```python
from build123d import *

# Parameters (mm, degrees)
SKETCH1_R           = 55
SKETCH1_R_2         = 41.4175
BOSS_EXTRUDE1_DEPTH = 15
CUT_EXTRUDE1_DEPTH  = 80.214897589
CUT_EXTRUDE2_START  = -10
CUT_EXTRUDE2_DEPTH  = 10
SKETCH4_R           = 2.75
CUT_EXTRUDE3_DEPTH  = 84.858511792
FILLET2_R           = 2
CHAMFER2_SIZE       = 1
CHAMFER3_SIZE       = 1


with BuildPart() as part:
    # Sketch1 → Boss-Extrude1 (new body)
    with BuildSketch(Plane(origin=(0, 0, 0), x_dir=(1, 0, 0), z_dir=(0, 1, 0))):
        with Locations(Location((0, 0, 0), (0, 0, 270))):
            Circle(SKETCH1_R)
        with Locations(Location((0, 0, 0), (0, 0, 270))):
            Circle(SKETCH1_R_2, mode=Mode.SUBTRACT)
    extrude(amount=BOSS_EXTRUDE1_DEPTH)

    # Sketch2 → Cut-Extrude1 (cut, through all)
    with BuildSketch(Plane(origin=(0, 15, 0), x_dir=(1, 0, 0), z_dir=(0, 1, 0))):
        with BuildLine():
            Line((-2.5, 41.341979951), (-2.5, 54.94315244))
            ThreePointArc((-2.5, 54.94315244), (0, 55), (2.5, 54.94315244))
            Line((2.5, 54.94315244), (2.5, 41.341979951))
            ThreePointArc((2.5, 41.341979951), (0, 41.4175), (-2.5, 41.341979951))
        make_face()
    extrude(amount=-CUT_EXTRUDE1_DEPTH, mode=Mode.SUBTRACT)

    # Sketch3 → Cut-Extrude2 (cut)
    with BuildSketch(Plane(origin=(0, 15, 0), x_dir=(1, 0, 0), z_dir=(0, 1, 0)).offset(CUT_EXTRUDE2_START)):
        with BuildLine():
            Line((-6.5, 54.614558499), (-6.5, 44.614558499))
            Line((-6.5, 44.614558499), (-32.164284074, 44.614558499))
            ThreePointArc((-32.164284074, 44.614558499), (-19.96826772, 51.247129522), (-6.5, 54.614558499))
        make_face()
        with BuildLine():
            Line((6.5, 44.614558499), (32.164284074, 44.614558499))
            ThreePointArc((32.164284074, 44.614558499), (19.96826772, 51.247129522), (6.5, 54.614558499))
            Line((6.5, 54.614558499), (6.5, 44.614558499))
        make_face()
    extrude(amount=CUT_EXTRUDE2_DEPTH, mode=Mode.SUBTRACT)

    # Sketch4 → Cut-Extrude3 (cut, through all)
    with BuildSketch(Plane.ZY.offset(6.5)):
        with Locations((-49.614558499, 10)):
            Circle(SKETCH4_R)
    extrude(amount=-CUT_EXTRUDE3_DEPTH, mode=Mode.SUBTRACT)

    # Fillet2
    fillet2_edges = [part.edges().sort_by_distance(p)[0] for p in [
        (-19.332142037, 5, -44.614558499),
        (19.332142037, 5, -44.614558499),
    ]]
    fillet(fillet2_edges, radius=FILLET2_R)

    # Chamfer2
    chamfer2_edges = [part.edges().sort_by_distance(p)[0] for p in [
        (0, 0, 55),
        (0, 15, 55),
    ]]
    chamfer(chamfer2_edges, length=CHAMFER2_SIZE)

    # Chamfer3
    chamfer3_edges = [part.edges().sort_by_distance(p)[0] for p in [
        (-41.398615683, 0, 1.250570198),
        (41.398615683, 15, 1.250570198),
    ]]
    chamfer(chamfer3_edges, length=CHAMFER3_SIZE)


solid = part.part
```
Design review of the part built by this model. Coordinates are the model's own, in mm. A direction names the side the tool comes from. Coordinates: 2 decimals unless noted, no trailing zeros. Order: outer loops, then holes, each group sorted by start corner. A loop starts at its lowest first (then second) coordinate and runs counter-clockwise, first axis right, second up. Notation, with made-up numbers: (36.5, 17.25) - (88.5, 17.25) arc R35 cw to (88.5, 52.25) - close; hole circle Ø8 at (3, -6.75). An arc over 180 degrees is marked (long way). Answer in a Markdown table with one row per item.
(1) Consider section B-B on y = 10. State the section outline as (x, z) points (1 decimal), plus the area to 3 significant figures.
Checked values:
| item | result |
|---|---|
| outline | (-32.2, -44.6) - (-6.5, -44.6) - (-6.5, -46.9) - (-2.5, -46.9) - (-2.5, -41.3) arc R41.4 cw (long way) to (2.5, -41.3) - (2.5, -46.9) - (6.5, -46.9) - (6.5, -44.6) - (32.2, -44.6) arc R55 ccw (long way) to start; (-6.5, -54.6) arc R55 ccw to (-2.5, -54.9) - (-2.5, -52.4) - (-6.5, -52.4) - close; (2.5, -54.9) arc R55 ccw to (6.5, -54.6) - (6.5, -52.4) - (2.5, -52.4) - close |
| area | 3,680 mm^2 |
(2) Wall thickness on line 1 along X through (y, z) = (11, 0.5); line 2 along X through (y, z) = (9.5, -26.5); line 3 along Z through (x, y) = (-16.5, 4.5): over which ranges is each line inside the solid? List them lowest first. Write a range as from..to.
Checked values:
| item | result |
|---|---|
| line 1 | -55..-41.41, 41.41..55 |
| line 2 | -48.19..-31.83, 31.83..48.19 |
| line 3 | -52.47..-37.99, 37.99..52.47 |
(3) Consider section C-C on y = 3. State the section outline as (x, z) points (1 decimal).
Checked values:
| item | result |
|---|---|
| outline | (-2.5, -54.9) - (-2.5, -41.3) arc R41.4 cw (long way) to (2.5, -41.3) - (2.5, -54.9) arc R55 ccw (long way) to start |
(4) For faces 1 (the flat face through (-19, 11, -44.615)), 2 (the flat face through (19, 11, -44.615)), 3 (the flat face through (-16, 15, 40)), 4 (the flat face through (2.5, 8, -47)), list the 3-axis set-ups (+Z, -Z, +X, -X, +Y, -Y) from which the entire face can be reached by the end or side of a thin tool; tool diameter is ignored.
Checked values:
| item | result |
|---|---|
| face 1 | -Z, -X, +Y |
| face 2 | -Z, +X, +Y |
| face 3 | +Z, -Z, +X, -X, +Y |
| face 4 | -Z, +Y, -Y |
(5) Consider section A-A on z = 0. State the section outline as (x, y) points.
Checked values:
| item | result |
|---|---|
| outline | (-55, 1) - (-54, 0) - (-42.42, 0) - (-41.42, 1) - (-41.42, 14) - (-42.42, 15) - (-54, 15) - (-55, 14) - close; (41.42, 1) - (42.42, 0) - (54, 0) - (55, 1) - (55, 14) - (54, 15) - (42.42, 15) - (41.42, 14) - close |
(6) The part is to be moulded in two halves that separate along X. For faces 5 (the flat face through (-15, 5, -50)), 6 (the flat face through (-6.5, 12, -52)), 7 (the conical face through (1.928, 14.84, 54.125)), 8 (the flat face through (-2.5, 8, -47)), say which applies: released by +X, released by -X, zero draft, split by the parting line, or undercut.
Checked values:
| item | result |
|---|---|
| face 5 | zero draft |
| face 6 | released by -X |
| face 7 | split by the parting line |
| face 8 | undercut |
(7) Clearance check with flat-ended pins moving along their axes: pin 1 (6.5 mm diameter, centred on x = -20.5, y = 11.5, fed in from -Z); pin 2 (6.5 mm diameter, centred on y = 10, z = -49.61, fed in from +X); pin 3 (2.5 mm diameter, centred on x = 13.5, z = -51, fed in from +Y). State where each tip first meets the part, or that it passes through.
Checked values:
| item | result |
|---|---|
| pin 1 | z = -44.61 |
| pin 2 | x = 6.5 |
| pin 3 | y = 5 |
